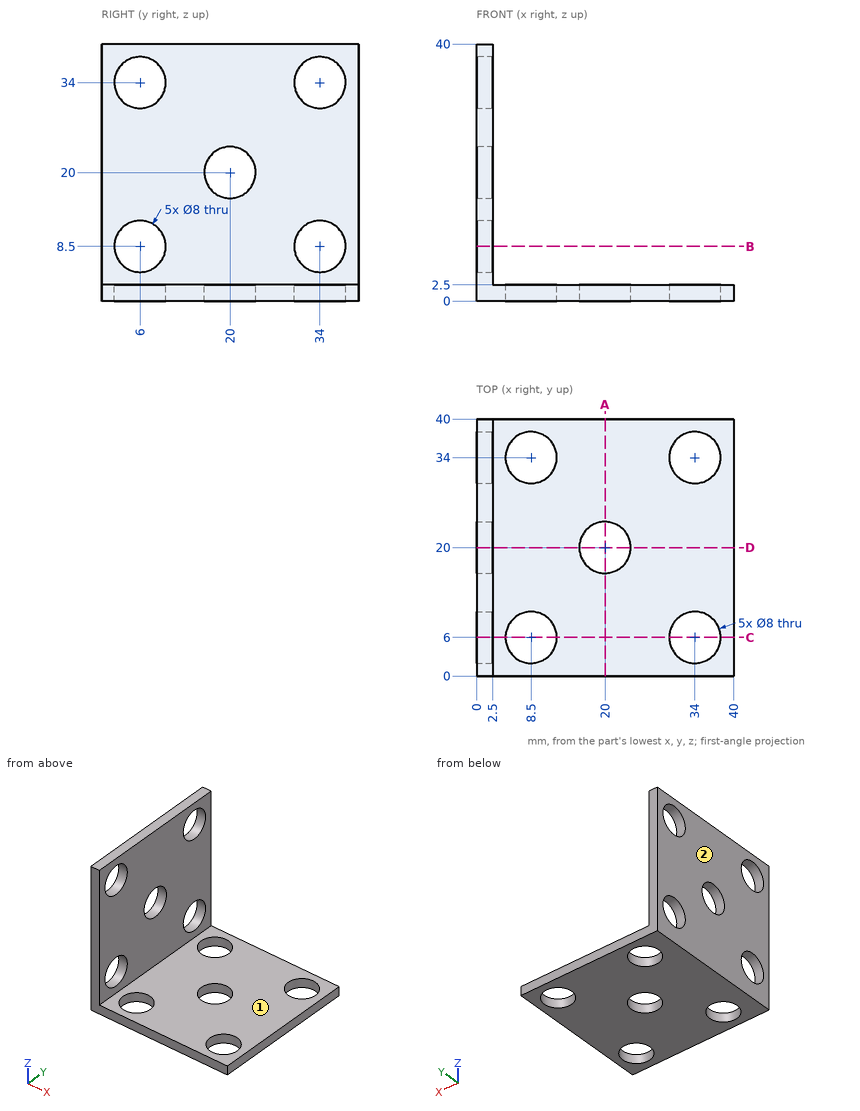
The figure shows three views and two pictorial views of one solid part (mm, origin at its lowest corner). Answer the questions. A direction names the side the tool comes from. Round coordinates to 2 decimals unless told otherwise and drop trailing zeros. Write each loop counter-clockwise with the first axis right and the second up, starting at its lowest first coordinate (ties: lowest second). Pieces come first, ordered by that corner, then holes. Notation, with made-up numbers: (83, 37) -> (127, 37) arc R16 ccw to (127, 41) -> close; hole circle Ø6 at (28, 43). An arc over 180 degrees is marked (long way). Answer as a JSON object with one key per item and string values. Group by question number.
Q1. Section B-B (z = 8.5) is taken. Write down the section's boundary in (x, y).
Q2. Straight lines are drawn through the part: line 1 along Z through (x, y) = (1, 34); line 2 along Y through (x, z) = (1.25, 8.5); line 3 along Z through (x, y) = (0.75, 20). For each, find the intervals that lie inside material, in ascending order.
Q3. Each of these flat-tipped pins is pushed along its axis until it touches: pin 1 Ø6.5 at (y, z) = (34, 34) entering from -X; pin 2 Ø13 at (x, y) = (34, 34) entering from +Z; pin 3 Ø1.5 at (y, z) = (11, 17) entering from +X. Where does it stop, or does it pass through?
Q4. Section D-D (y = 20) is taken. Write down the section's boundary in (x, z).
Q5. Section A-A (x = 20) is taken. Write down the section's boundary in (y, z).
Q6. Section C-C (y = 6) is taken. Write down the section's boundary in (x, z).
Q7. Which of the six approach directions +Z, -Z, +X, -X, +Y, -Y give full straight-line access (tool end or side, diameter ignored) to the marked faces 1 and 2?
Check values:
{
 "1": {"outline": "(0, 0) -> (2.5, 0) -> (2.5, 2) -> (0, 2) -> close; (0, 10) -> (2.5, 10) -> (2.5, 30) -> (0, 30) -> close; (0, 38) -> (2.5, 38) -> (2.5, 40) -> (0, 40) -> close"},
 "2": {"line 1": "0 to 4.5, 12.5 to 30, 38 to 40", "line 2": "0 to 2, 10 to 30, 38 to 40", "line 3": "0 to 16, 24 to 40"},
 "3": {"pin 1": "through", "pin 2": "z = 2.5", "pin 3": "x = 2.5"},
 "4": {"outline": "(0, 0) -> (16, 0) -> (16, 2.5) -> (2.5, 2.5) -> (2.5, 16) -> (0, 16) -> close; (0, 24) -> (2.5, 24) -> (2.5, 40) -> (0, 40) -> close; (24, 0) -> (40, 0) -> (40, 2.5) -> (24, 2.5) -> close"},
 "5": {"outline": "(0, 0) -> (16, 0) -> (16, 2.5) -> (0, 2.5) -> close; (24, 0) -> (40, 0) -> (40, 2.5) -> (24, 2.5) -> close"},
 "6": {"outline": "(0, 0) -> (4.5, 0) -> (4.5, 2.5) -> (2.5, 2.5) -> (2.5, 4.5) -> (0, 4.5) -> close; (0, 12.5) -> (2.5, 12.5) -> (2.5, 30) -> (0, 30) -> close; (0, 38) -> (2.5, 38) -> (2.5, 40) -> (0, 40) -> close; (12.5, 0) -> (30, 0) -> (30, 2.5) -> (12.5, 2.5) -> close; (38, 0) -> (40, 0) -> (40, 2.5) -> (38, 2.5) -> close"},
 "7": {"face 1": "+Z, +X, +Y, -Y", "face 2": "+Z, -Z, -X, +Y, -Y"}
}
